The figure shows three views and two pictorial views of one solid part (mm, origin at its lowest corner). Answer the questions. Give positions to 0.01 mm unless a question says otherwise; leave off trailing zeros. Order: outer loops, then holes, each group sorted by start corner. A loop starts at its lowest first (then second) coordinate and runs counter-clockwise, first axis right, second up. Notation, with made-up numbers: (-28.5, -22) - (25.5, -22) arc R20 cw to (25.5, -15) - close; hole circle Ø7 at (20.5, 78.25). An arc over 180 degrees is marked (long way). Answer as a JSON object with one key per item and string values. Group by question number.
Q1. Consider line 1 (Y direction, x = 5, z = 7.25); line 2 (X direction, y = 30.5, z = 1); line 3 (Y direction, x = 38, z = 5.5). Determine where each line is inside the solid, lowest interval first.
Q2. A cutting plane is placed at C-C, the plane y = 27.5. Give the vertices of the cut face in (x, z).
Q3. The mould has two halves that part along Y. Classify the marked faces 1, 2, 3 and 4: released by +Y, released by -Y, zero draft, split by the parting line, or undercut.
Q4. A cutting plane is placed at D-D, the plane x = 21. Give the vertices of the cut face in (y, z), and give its area (4 significant figures).
Q5. Given pin 1 (2.5 mm diameter, centred on x = 44, y = 27.5, fed in from +Z); pin 2 (1 mm diameter, centred on x = 0.5, y = 6, fed in from +Z); pin 3 (5 mm diameter, centred on x = 74.5, z = 3, fed in from +Y), each flat-ended and moving along its own axis, determine where each tip first touches the part or whether it passes through.
Q6. A cutting plane is placed at A-A, the plane z = 1.5. Give the vertices of the cut face in (x, y), and give its area (3 significant figures).
Q7. A cutting plane is placed at B-B, the plane x = 71. Give the vertices of the cut face in (y, z).
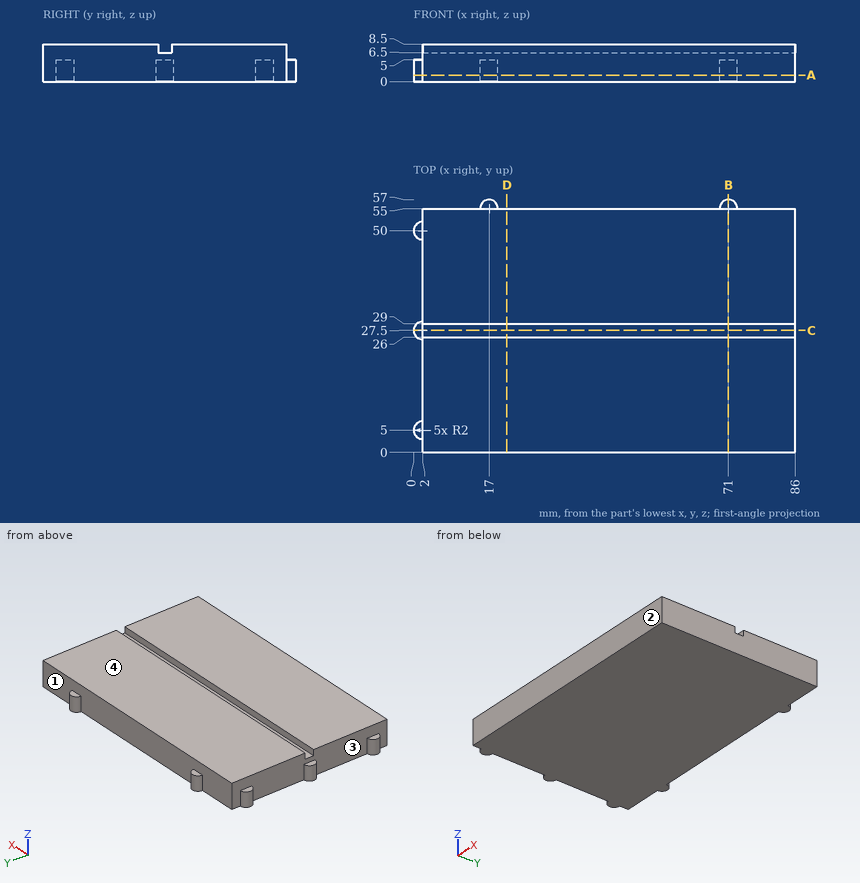
Reply:
{
 "1": {"line 1": "y = 0 to 26, 29 to 55", "line 2": "x = 2 to 86", "line 3": "y = 0 to 55"},
 "2": {"outline": "(0, 0) - (86, 0) - (86, 6.5) - (2, 6.5) - (2, 5) - (0, 5) - close"},
 "3": {"face 1": "released by +Y", "face 2": "released by -Y", "face 3": "undercut", "face 4": "zero draft"},
 "4": {"outline": "(0, 0) - (55, 0) - (55, 8.5) - (29, 8.5) - (29, 6.5) - (26, 6.5) - (26, 8.5) - (0, 8.5) - close", "area": "461.5 mm^2"},
 "5": {"pin 1": "stops at z = 6.5", "pin 2": "stops at z = 5", "pin 3": "stops at y = 56.73"},
 "6": {"outline": "(2, 0) - (86, 0) - (86, 55) - (73, 55) arc R2 ccw to (69, 55) - (19, 55) arc R2 ccw to (15, 55) - (2, 55) - (2, 52) arc R2 ccw to (2, 48) - (2, 29.5) arc R2 ccw to (2, 25.5) - (2, 7) arc R2 ccw to (2, 3) - close", "area": "4,650 mm^2"},
 "7": {"outline": "(0, 0) - (57, 0) - (57, 5) - (55, 5) - (55, 8.5) - (29, 8.5) - (29, 6.5) - (26, 6.5) - (26, 8.5) - (0, 8.5) - close"}
}
